The model under review builds one solid part; all positions refer to its coordinate system, in mm. A direction names the side the tool comes from. Coordinates: 2 decimals unless noted, no trailing zeros. Write each loop counter-clockwise with the first axis right and the second up, starting at its lowest first coordinate (ties: lowest second). Pieces come first, ordered by that corner, then holes. Notation, with made-up numbers: (-1.5, 61) - (18.5, 61) arc R30 cw to (18.5, 89) - close; hole circle Ø10 at (63, 31). An arc over 180 degrees is marked (long way). Put each result on its own line as item: value.
from build123d import *

# Parameters (mm, degrees)
SKETCH1_W                      = 68
SKETCH1_H                      = 48
BOSS_EXTRUDE1_DEPTH            = 35
SHELL1_T                       = -2
FILLET1_R                      = 5
FILLET2_R                      = 3
CUT_EXTRUDE1_REACH             = 80.467
CUT_EXTRUDE1_DIRECTION_2_REACH = 80.467
CUT_EXTRUDE2_DEPTH             = 55.378304497
CUT_EXTRUDE2_DEPTH_BACK        = 55.378304497
SKETCH3_R                      = 2.5
FILLET3_R                      = 5
SKETCH4_R                      = 4
CUT_EXTRUDE3_DEPTH             = 55.378304497


with BuildPart() as part:
    # Sketch1 → Boss-Extrude1 (new body)
    with BuildSketch(Plane(origin=(0, 0, 0), x_dir=(1, 0, 0), z_dir=(0, 1, 0))):
        Rectangle(SKETCH1_W, SKETCH1_H)
    extrude(amount=BOSS_EXTRUDE1_DEPTH)

    # Shell1
    shell1_openings = [part.faces().sort_by_distance(p)[0] for p in [
        (0, 0, 0),
    ]]
    offset(amount=SHELL1_T, openings=shell1_openings, kind=Kind.INTERSECTION)

    # Fillet1
    fillet1_edges = [part.edges().sort_by_distance(p)[0] for p in [
        (0, 35, 24),
        (0, 35, -24),
    ]]
    fillet(fillet1_edges, radius=FILLET1_R)

    # Fillet2
    fillet2_edges = [part.edges().sort_by_distance(p)[0] for p in [
        (0, 33, -22),
        (0, 33, 22),
    ]]
    fillet(fillet2_edges, radius=FILLET2_R)

    # Sketch2 → Cut-Extrude1 (cut, up to next)
    with BuildSketch(Plane(origin=(-32, 0, 0), x_dir=(0, 0, -1), z_dir=(1, 0, 0)), mode=Mode.PRIVATE) as cut_extrude1_sk1:
        with BuildLine():
            Line((22, 0), (22, 30))
            ThreePointArc((22, 30), (21.121320344, 32.121320344), (19, 33))
            Line((19, 33), (-19, 33))
            ThreePointArc((-19, 33), (-21.121320344, 32.121320344), (-22, 30))
            Line((-22, 30), (-22, 0))
            Line((-22, 0), (22, 0))
        make_face()
    cut_extrude1_tool1 = extrude(cut_extrude1_sk1.sketch, amount=-CUT_EXTRUDE1_REACH, mode=Mode.PRIVATE) & part.part
    add(cut_extrude1_tool1.solids().sort_by_distance((-32, 16.457775, 0))[0], mode=Mode.SUBTRACT)

    # Sketch2 → Cut-Extrude1 direction 2 (cut, up to next)
    with BuildSketch(Plane(origin=(-32, 0, 0), x_dir=(0, 0, -1), z_dir=(1, 0, 0)), mode=Mode.PRIVATE) as cut_extrude1_direction_2_sk1:
        with BuildLine():
            Line((22, 0), (22, 30))
            ThreePointArc((22, 30), (21.121320344, 32.121320344), (19, 33))
            Line((19, 33), (-19, 33))
            ThreePointArc((-19, 33), (-21.121320344, 32.121320344), (-22, 30))
            Line((-22, 30), (-22, 0))
            Line((-22, 0), (22, 0))
        make_face()
    cut_extrude1_direction_2_tool1 = extrude(cut_extrude1_direction_2_sk1.sketch, amount=CUT_EXTRUDE1_DIRECTION_2_REACH, mode=Mode.PRIVATE) & part.part
    add(cut_extrude1_direction_2_tool1.solids().sort_by_distance((-32, 16.457775, 0))[0], mode=Mode.SUBTRACT)

    # Sketch3 → Cut-Extrude2 (cut, two sides: drawn at the far end of the back side and taken through both)
    with BuildSketch(Plane.XY.offset(-CUT_EXTRUDE2_DEPTH_BACK)):
        with Locations((-15, 10)):
            Circle(SKETCH3_R)
        with Locations((15, 10)):
            Circle(SKETCH3_R)
    extrude(amount=CUT_EXTRUDE2_DEPTH + CUT_EXTRUDE2_DEPTH_BACK, mode=Mode.SUBTRACT)

    # Fillet3
    fillet3_edges = [part.edges().sort_by_distance(p)[0] for p in [
        (-34, 0, -23),
        (34, 0, -23),
        (-34, 0, 23),
        (34, 0, 23),
    ]]
    fillet(fillet3_edges, radius=FILLET3_R)

    # Sketch4 → Cut-Extrude3 (cut, through all)
    with BuildSketch(Plane(origin=(0, 35, 0), x_dir=(1, 0, 0), z_dir=(0, 1, 0))):
        with Locations(Location((0, 0, 0), (0, 0, 270))):
            Circle(SKETCH4_R)
    extrude(amount=-CUT_EXTRUDE3_DEPTH, mode=Mode.SUBTRACT)


solid = part.part
1. Machinability: for faces 1 (the flat face through (0, 15, -24)), 2 (the cylindrical face through (0.48, 32.1, 21.14)), which of the approach directions +Z, -Z, +X, -X, +Y, -Y give a long, thin tool a straight path to every point of the face, cutting with its end or side? Answer none if there is none.
Determined:
face 1: -Z, +X, -X, +Y, -Y
face 2: +X, -X, -Y
2. Consider section A-A on z = 0. State the section outline as (x, y) points, plus the area to 3 significant figures.
Determined:
outline: (-34, 33) - (-4, 33) - (-4, 35) - (-34, 35) - close; (4, 33) - (34, 33) - (34, 35) - (4, 35) - close
area: 120 mm^2
3. Consider section C-C on y = 24.5. State the section outline as (x, z) points.
Determined:
outline: (-34, -24) - (34, -24) - (34, -22) - (-34, -22) - close; (-34, 22) - (34, 22) - (34, 24) - (-34, 24) - close
4. For pin 1 Ø6 at (y, z) = (20.5, -16.5) entering from +X; pin 2 Ø11.5 at (x, z) = (3, 1) entering from -Y, all flat-tipped, find the tip position at first contact; note any pin that passes through.
Determined:
pin 1: passes through
pin 2: stops at y = 33
5. Consider section D-D on x = 0. State the section outline as (y, z) points, plus the area to 3 significant figures.
Determined:
outline: (0, -24) - (30, -24) arc R5 ccw to (35, -19) - (35, -4) - (33, -4) - (33, -19) arc R3 cw to (30, -22) - (0, -22) - close; (0, 22) - (30, 22) arc R3 cw to (33, 19) - (33, 4) - (35, 4) - (35, 19) arc R5 ccw to (30, 24) - (0, 24) - close
area: 205 mm^2
6. The part is to be moulded in two halves that separate along Y. For faces 3 (the flat face through (-34, 33.3, 0.1)), 4 (the cylindrical face through (0, 33, -23)), 5 (the cylindrical face through (13, 8.5, -23)), say which applies: +Y half, -Y half, draft (parallel to the pull), parting line (faces both ways), or undercut.
Determined:
face 3: draft
face 4: +Y half
face 5: undercut
7. Consider section B-B on x = -15. State the section outline as (y, z) points.
Determined:
outline: (0, -24) - (7.5, -24) - (7.5, -22) - (0, -22) - close; (0, 22) - (7.5, 22) - (7.5, 24) - (0, 24) - close; (12.5, -24) - (30, -24) arc R5 ccw to (35, -19) - (35, 19) arc R5 ccw to (30, 24) - (12.5, 24) - (12.5, 22) - (30, 22) arc R3 cw to (33, 19) - (33, -19) arc R3 cw to (30, -22) - (12.5, -22) - close
8. To check wall thickness, follow probe 1 along X at (y, z) = (10, -23.2); probe 2 along Y at (x, z) = (15, 23); probe 3 along Z at (x, y) = (30.5, 13). State the ranges of each line that lie inside material, in increasing order.
Determined:
probe 1: x = -34 to -17.5, -12.5 to 12.5, 17.5 to 34
probe 2: y = 0 to 7.5, 12.5 to 33
probe 3: z = -24 to -22, 22 to 24
